from build123d import *

# Parameters (mm, degrees)
ESBO_O1_R                = 12.5
RESSALTO_EXTRUS_O1_DEPTH = 112.9
ESBO_O2_R                = 10
RESSALTO_EXTRUS_O2_DEPTH = 27.1
ESBO_O3_R                = 7.5
CORTE_EXTRUS_O1_DEPTH    = 142.111657917
ESBO_O5_R                = 5
CORTE_EXTRUS_O2_DEPTH    = 15


with BuildPart() as part:
    # Esboço1 → Ressalto-extrusão1 (new body)
    with BuildSketch(Plane(origin=(0, 0, 0), x_dir=(1, 0, 0), z_dir=(0, 1, 0))):
        with Locations(Location((0, 0, 0), (0, 0, 90))):
            Circle(ESBO_O1_R)
    extrude(amount=RESSALTO_EXTRUS_O1_DEPTH)

    # Esboço2 → Ressalto-extrusão2 (add)
    with BuildSketch(Plane(origin=(0, 112.9, 0), x_dir=(1, 0, 0), z_dir=(0, 1, 0))):
        with Locations(Location((0, 0, 0), (0, 0, 90))):
            Circle(ESBO_O2_R)
    extrude(amount=RESSALTO_EXTRUS_O2_DEPTH)

    # Esboço3 → Corte-extrusão1 (cut, through all)
    with BuildSketch(Plane(origin=(0, 140, 0), x_dir=(1, 0, 0), z_dir=(0, 1, 0))):
        with Locations(Location((0, 0, 0), (0, 0, 270))):
            Circle(ESBO_O3_R)
    extrude(amount=-CORTE_EXTRUS_O1_DEPTH, mode=Mode.SUBTRACT)

    # Esboço5 → Corte-extrusão2 (cut, symmetric)
    with BuildSketch(Plane(origin=(0, 0, 0), x_dir=(0, 0, -1), z_dir=(1, 0, 0))):
        with Locations((0, 28)):
            Circle(ESBO_O5_R)
    extrude(amount=CORTE_EXTRUS_O2_DEPTH, both=True, mode=Mode.SUBTRACT)


solid = part.part
Check sheet for the modelled part. Datum: model origin and axes. Units: mm. A direction names the side the tool comes from. Round coordinates to 2 decimals unless told otherwise and drop trailing zeros. Loops run counter-clockwise (first coordinate to the right, second up) from the corner with the lowest first, then second, coordinate; pieces in that order, holes last. Notation, with made-up numbers: M 2.5,52 L 39.5,52 A24 ccw 39.5,81 Z; hole C 69,-24.75 d11. An arc over 180 degrees is marked long. One line per item, written item: value.
(1) Depth check by flat-ended pin: pin 1 Ø2 at (x, z) = (-9.5, -8) entering from +Y; pin 2 Ø8 at (y, z) = (28, 0) entering from +X; pin 3 Ø7.5 at (x, z) = (3, 5.5) entering from +Y; pin 4 Ø6 at (y, z) = (89.5, -8.5) entering from -X (3 decimals). Enter the tip coordinate at first touch or a pass-through.
Computed values:
pin 1: stops at y = 112.9
pin 2: passes through
pin 3: stops at y = 140
pin 4: stops at x = -11.225
(2) Sectioned sample at D-D, the plane y = 9. Record the cut outline in (x, z), then the cut area to 3 significant figures.
Computed values:
outline: C 0,0 d25; hole C 0,0 d15
area: 314 mm^2
(3) Release check for a two-part mould opening along Z. For faces 1 (the face through (9.097, 26.085, -4.619)), 2 (the face through (-7, 140, -4)), 3 (the face through (-9, 23.564, -2.307)), 4 (the face through (9.76, 126.26, 2.17)) record: +Z half, -Z half, draft (parallel to the pull), parting line (faces both ways), or undercut.
Computed values:
face 1: undercut
face 2: draft
face 3: undercut
face 4: parting line
(4) Sectioned sample at C-C, the plane y = 30.5. Record the cut outline in (x, z).
Computed values:
outline: M -11.73,-4.33 A12.5 ccw 11.73,-4.33 L 6.12,-4.33 A7.5 cw -6.12,-4.33 Z; M -11.73,4.33 L -6.12,4.33 A7.5 cw 6.12,4.33 L 11.73,4.33 A12.5 ccw Z
(5) Thickness scan on line 1 (X direction, y = 42.5, z = 0); line 2 (Y direction, x = 9, z = 0); line 3 (X direction, y = 13.5, z = 6). Record the ranges inside material, lowest first.
Computed values:
line 1: x = -12.5 to -7.5, 7.5 to 12.5
line 2: y = 0 to 23, 33 to 140
line 3: x = -10.97 to -4.5, 4.5 to 10.97
(6) Sectioned sample at A-A, the plane z = 0. Record the cut outline in (x, y), then the cut area to 3 significant figures.
Computed values:
outline: M -12.5,0 L -7.5,0 L -7.5,23 L -12.5,23 Z; M -12.5,33 L -7.5,33 L -7.5,140 L -10,140 L -10,112.9 L -12.5,112.9 Z; M 7.5,0 L 12.5,0 L 12.5,23 L 7.5,23 Z; M 7.5,33 L 12.5,33 L 12.5,112.9 L 10,112.9 L 10,140 L 7.5,140 Z
area: 1,160 mm^2
(7) Access from +Z, -Z, +X, -X, +Y, -Y to the whole of each face (thin tool, end or side, straight path). Record for faces 5 (the face through (8, 0, 0)), 6 (the face through (-10.2, 112.9, 0.1)).
Computed values:
face 5: +Z, -Z, +X, -X, -Y
face 6: +Y
(8) Sectioned sample at B-B, the plane x = 0. Record the cut outline in (y, z).
Computed values:
outline: M 0,-12.5 L 112.9,-12.5 L 112.9,-10 L 140,-10 L 140,-7.5 L 0,-7.5 Z; M 0,7.5 L 140,7.5 L 140,10 L 112.9,10 L 112.9,12.5 L 0,12.5 Z
